```python
from build123d import *

# Parameters (mm, degrees)
EXTRUDE_1_DEPTH          = 56
CUT_EXTRUDE_1_DEPTH      = 85.687661439
CUT_EXTRUDE_1_DEPTH_BACK = 85.687661439
SKETCH_2_R               = 3.25
CUT_EXTRUDE_2_DEPTH      = 88.3842091
CUT_EXTRUDE_2_DEPTH_BACK = 88.3842091
SKETCH_3_R               = 3.25


with BuildPart() as part:
    # 草图1 → 凸台-拉伸1 (new body)
    with BuildSketch(Plane(origin=(0, 0, 0), x_dir=(1, 0, 0), z_dir=(0, 1, 0))):
        Polygon((0, 0), (-30, 0), (-30, 4), (-4, 4), (-4, 60), (0, 60), align=None)
    extrude(amount=EXTRUDE_1_DEPTH)

    # 草图2 → 切除-拉伸1 (cut, two sides: drawn at the far end of the back side and taken through both)
    with BuildSketch(Plane(origin=(0, 0, -4), x_dir=(-1, 0, 0), z_dir=(0, 0, -1)).offset(-CUT_EXTRUDE_1_DEPTH_BACK)):
        with Locations((15, 43)):
            Circle(SKETCH_2_R)
        with Locations((15, 13)):
            Circle(SKETCH_2_R)
    extrude(amount=CUT_EXTRUDE_1_DEPTH + CUT_EXTRUDE_1_DEPTH_BACK, mode=Mode.SUBTRACT)

    # 草图3 → 切除-拉伸2 (cut, two sides: drawn at the far end of the back side and taken through both)
    with BuildSketch(Plane(origin=(0, 0, 0), x_dir=(0, 0, -1), z_dir=(1, 0, 0)).offset(-CUT_EXTRUDE_2_DEPTH_BACK)):
        with Locations((15, 41)):
            Circle(SKETCH_3_R)
        with Locations((15, 15)):
            Circle(SKETCH_3_R)
        with Locations((45, 15)):
            Circle(SKETCH_3_R)
        with Locations((45, 41)):
            Circle(SKETCH_3_R)
    extrude(amount=CUT_EXTRUDE_2_DEPTH + CUT_EXTRUDE_2_DEPTH_BACK, mode=Mode.SUBTRACT)


solid = part.part
```
Part model, mm, in its own coordinate system. A direction names the side the tool comes from. Round coordinates to 2 decimals unless told otherwise and drop trailing zeros. Write each loop counter-clockwise with the first axis right and the second up, starting at its lowest first coordinate (ties: lowest second). Pieces come first, ordered by that corner, then holes. Notation, with made-up numbers: (10.5, 37) -> (65.5, 37) arc R11 cw to (65.5, 44) -> close; hole circle Ø7 at (48.25, 73.5). An arc over 180 degrees is marked (long way). Return JSON: item names as keys, results as strings. Group by question number.
Q1. Pin check, flat tips, straight feed: pin 1 (4 mm diameter, centred on y = 13, z = -14.5, fed in from -X); pin 2 (5 mm diameter, centred on y = 15, z = -15, fed in from +X); pin 3 (10.5 mm diameter, centred on x = -15, y = 43, fed in from +Z); pin 4 (10 mm diameter, centred on x = -25.5, y = 10.5, fed in from -Z). Stop position of each tip, or through.
Q2. Which spindle directions (+Z, -Z, +X, -X, +Y, -Y) get a long thin tool onto all of the face, cutting with end or side? Do faces 4 (the cylindrical face through (-2.03, 15.98, -48.1)), 5 (the flat face through (-17, 28, -4)). Say none if no direction does.
Q3. Probe L1, parallel to Y at x = -15, z = -2.05; L2, parallel to Y at x = -0.95, z = -45; L3, parallel to Z at x = -1.45, y = 41. List the from-to ranges inside material, lowest first. Write a range as [from, to].
Q4. Saw through at B-B on z = -15. Write the cut outline in (x, y).
Q5. Saw through at D-D on x = -10.5. Write the cut outline in (y, z), plus the area to 3 significant figures.
Q6. Saw through at A-A on y = 41. Write the cut outline in (x, z), plus the area to 3 significant figures.
Q7. Mould opens along Z. For faces 1 (the flat face through (-2, 28, -60)), 2 (the cylindrical face through (-11.753, 13.143, -1.972)), 3 (the cylindrical face through (-2.028, 18.222, -14.577)) say: pulls with the +Z half, pulls with the -Z half, needs draft (parallel to the pull), parting line crosses it, or undercut.
Q8. Saw through at C-C on y = 17. Write the cut outline in (x, z), plus the area to 3 significant figures.
Answer:
{
 "1": {"pin 1": "x = -4", "pin 2": "through", "pin 3": "z = 0", "pin 4": "z = -4"},
 "2": {"face 4": "+X, -X", "face 5": "-Z, -X, +Y, -Y"},
 "3": {"L1": "[0, 9.75], [16.25, 39.75], [46.25, 56]", "L2": "[0, 11.75], [18.25, 37.75], [44.25, 56]", "L3": "[-60, -48.25], [-41.75, -18.25], [-11.75, 0]"},
 "4": {"outline": "(-4, 0) -> (0, 0) -> (0, 11.75) -> (-4, 11.75) -> close; (-4, 18.25) -> (0, 18.25) -> (0, 37.75) -> (-4, 37.75) -> close; (-4, 44.25) -> (0, 44.25) -> (0, 56) -> (-4, 56) -> close"},
 "5": {"outline": "(0, -4) -> (56, -4) -> (56, 0) -> (0, 0) -> close", "area": "224 mm2"},
 "6": {"outline": "(-30, -4) -> (-17.56, -4) -> (-17.56, 0) -> (-30, 0) -> close; (-12.44, -4) -> (-4, -4) -> (-4, -11.75) -> (0, -11.75) -> (0, 0) -> (-12.44, 0) -> close; (-4, -60) -> (0, -60) -> (0, -48.25) -> (-4, -48.25) -> close; (-4, -41.75) -> (0, -41.75) -> (0, -18.25) -> (-4, -18.25) -> close", "area": "272 mm2"},
 "7": {"face 1": "pulls with the -Z half", "face 2": "needs draft", "face 3": "undercut"},
 "8": {"outline": "(-30, -4) -> (-4, -4) -> (-4, -12.44) -> (0, -12.44) -> (0, 0) -> (-30, 0) -> close; (-4, -60) -> (0, -60) -> (0, -47.56) -> (-4, -47.56) -> close; (-4, -42.44) -> (0, -42.44) -> (0, -17.56) -> (-4, -17.56) -> close", "area": "303 mm2"}
}
